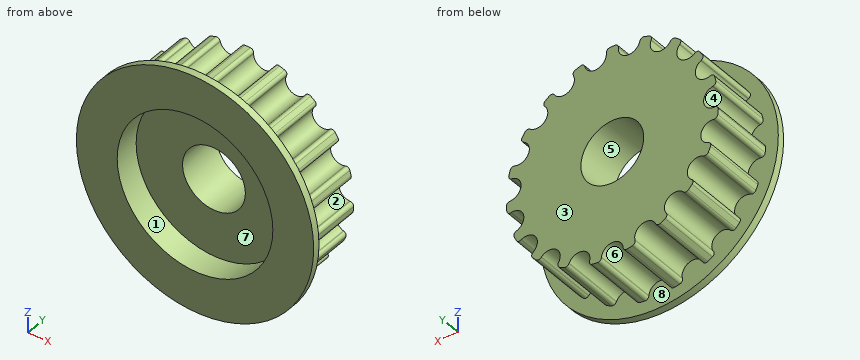
from build123d import *

# Parameters (mm, degrees)
SKETCH_1_R                       = 17
EXTRUDE_1_DEPTH                  = 4.01
SKETCH_3_R                       = 15.205
EXTRUDE_2_DEPTH                  = 9
SKETCH_4_R                       = 4.5
CUT_EXTRUDE_2_DEPTH              = 14.01
CUT_EXTRUDE_4_DEPTH              = 9
FILLET_2_R                       = 0.5
PATTERN_CIRCULAR_7_COUNT         = 19
FILLET_2_OF_PATTERN_CIRCULAR_7_R = 0.5
CUT_EXTRUDE_START                = -3
SKETCH_2_R                       = 11.05
CUT_EXTRUDE_5_DEPTH              = 3
SKETCH_6_R                       = 17
CUT_EXTRUDE_6_DEPTH              = 3
SKETCH_7_R                       = 11.15
CUT_EXTRUDE_7_DEPTH              = 3.6


with BuildPart() as part:
    # Sketch 1 → Extrude 1 (new body)
    with BuildSketch(Plane(origin=(0, 0, 0), x_dir=(1, 0, 0), z_dir=(0, 1, 0))):
        Circle(SKETCH_1_R)
    extrude(amount=EXTRUDE_1_DEPTH)

    # Sketch 3 → Extrude 2 (add)
    with BuildSketch(Plane(origin=(0, 4.01, 0), x_dir=(1, 0, 0), z_dir=(0, 1, 0))):
        Circle(SKETCH_3_R)
    extrude(amount=EXTRUDE_2_DEPTH)

    # Sketch 4 → Cut-Extrude 2 (cut, through all)
    with BuildSketch(Plane(origin=(0, 13.01, 0), x_dir=(1, 0, 0), z_dir=(0, 1, 0))):
        Circle(SKETCH_4_R)
    extrude(amount=-CUT_EXTRUDE_2_DEPTH, mode=Mode.SUBTRACT)

    # Sketch 5 → Cut-Extrude 4 (cut)
    with BuildSketch(Plane(origin=(0, 13.01, 0), x_dir=(1, 0, 0), z_dir=(0, 1, 0))):
        with BuildLine():
            Line((-1.615240041, 15.118962418), (-1.551172735, 14.519279917))
            ThreePointArc((-1.551172735, 14.519279917), (-2e-09, 13.125), (1.551172735, 14.519279913))
            Line((1.551172735, 14.519279913), (1.615240041, 15.118962418))
            ThreePointArc((1.615240041, 15.118962418), (0, 15.205), (-1.615240041, 15.118962418))
        make_face()
    cut_extrude_4 = extrude(amount=-CUT_EXTRUDE_4_DEPTH, mode=Mode.SUBTRACT)

    # Fillet 2
    fillet_2_edges = [part.edges().sort_by_distance(p)[0] for p in [
        (-1.615240041, 8.51, -15.118962418),
        (1.615240041, 8.51, -15.118962418),
    ]]
    fillet(fillet_2_edges, radius=FILLET_2_R)

    # Pattern Circular 7: Cut-Extrude 4 ×19 about axis
    pattern_circular_7_axis = Axis((0, 0, 0), (0, 1, 0))
    for i in range(1, PATTERN_CIRCULAR_7_COUNT):
        add(cut_extrude_4.rotate(pattern_circular_7_axis, i * 360 / PATTERN_CIRCULAR_7_COUNT), mode=Mode.SUBTRACT)

    # Fillet 2 of Pattern Circular 7
    fillet_2_of_pattern_circular_7_edges = [part.edges().sort_by_distance(p)[0] for p in [
        (-6.436840952, 8.51, -13.775307748),
        (-3.381397192, 8.51, -14.824242916),
        (-10.560910269, 8.51, -10.938884737),
        (-8.011607571, 8.51, -12.923086672),
        (-13.540541088, 8.51, -6.917063831),
        (-11.773635958, 8.51, -9.621513464),
        (-15.052844177, 8.51, -2.145671729),
        (-14.259808201, 8.51, -5.27729998),
        (-14.933938031, 8.51, 2.858237198),
        (-15.200708962, 8.51, -0.361209156),
        (-13.196707975, 8.51, 7.552411775),
        (-14.494377044, 8.51, 4.594024283),
        (-10.029409842, 8.51, 11.428165348),
        (-12.217354469, 8.51, 9.051423909),
        (-5.775269531, 8.51, 14.065499879),
        (-8.616391966, 8.51, 12.527961306),
        (-0.895289153, 8.51, 15.17861925),
        (-4.081709697, 8.51, 14.646899704),
        (4.081709697, 8.51, 14.646899704),
        (0.895289153, 8.51, 15.17861925),
        (8.616391966, 8.51, 12.527961306),
        (5.775269531, 8.51, 14.065499879),
        (12.217354469, 8.51, 9.051423909),
        (10.029409842, 8.51, 11.428165348),
        (14.494377044, 8.51, 4.594024283),
        (13.196707975, 8.51, 7.552411775),
        (15.200708962, 8.51, -0.361209156),
        (14.933938031, 8.51, 2.858237198),
        (14.259808201, 8.51, -5.27729998),
        (15.052844177, 8.51, -2.145671729),
        (11.773635958, 8.51, -9.621513464),
        (13.540541088, 8.51, -6.917063831),
        (8.011607571, 8.51, -12.923086672),
        (10.560910269, 8.51, -10.938884737),
        (3.381397192, 8.51, -14.824242916),
        (6.436840952, 8.51, -13.775307748),
    ]]
    fillet(fillet_2_of_pattern_circular_7_edges, radius=FILLET_2_OF_PATTERN_CIRCULAR_7_R)

    # Sketch 2 → Cut-Extrude 5 (cut)
    with BuildSketch(Plane.XZ.offset(CUT_EXTRUDE_START)):
        Circle(SKETCH_2_R)
    extrude(amount=CUT_EXTRUDE_5_DEPTH, mode=Mode.SUBTRACT)

    # Sketch 6 → Cut-Extrude 6 (cut)
    with BuildSketch(Plane.XZ):
        Circle(SKETCH_6_R)
    extrude(amount=-CUT_EXTRUDE_6_DEPTH, mode=Mode.SUBTRACT)

    # Sketch 7 → Cut-Extrude 7 (cut)
    with BuildSketch(Plane.XZ.offset(-3)):
        Circle(SKETCH_7_R)
    extrude(amount=-CUT_EXTRUDE_7_DEPTH, mode=Mode.SUBTRACT)


solid = part.part
Could you check a few things on this model? Use its own coordinates, in mm. Face numbers are marked on the shaded views. A direction names the side the tool comes from. Give positions to 0.01 mm unless a question says otherwise; leave off trailing zeros. Order: outer loops, then holes, each group sorted by start corner. A loop starts at its lowest first (then second) coordinate and runs counter-clockwise, first axis right, second up.
1. Will these pins go through, and if not, where does the flat tip stop? P1, Ø1, axis at x = -5.5, y = 7.5, coming from the +Z side; P2, Ø18, axis at x = 0, z = 0, coming from the +Y side; P3, Ø6, axis at y = 11.5, z = 1, coming from the +X side; P4, Ø1, axis at x = -11, y = 5.5, coming from the +Z side.
2. We'd pull the mould along X, two halves only. Please class the marked faces 1, 2 and 3: pulls with the +X half, pulls with the -X half, needs draft (parallel to the pull), parting line crosses it, or undercut.
3. I need wall thicknesses on L1, parallel to Z at x = 0, y = 4.5 (3 decimals); L2, parallel to X at y = 8, z = -13.5; L3, parallel to Y at x = -11, z = -0.5. Which ranges of each line are inside material? Lowest first, please.
4. For the marked faces 4, 5, 6, 7 and 8, which set-ups out of +Z, -Z, +X, -X, +Y, -Y let a thin tool reach every point of the face, with its end or its side?
5. Suppose I cut it at A-A (z = 5.5). List the corners of the cut face in (x, y) for me, plus the area to 3 significant figures.
Solved:
1. P1: stops at z = 14.36
1. P2: stops at y = 13.01
1. P3: stops at x = 15.18
1. P4: stops at z = 8.55
2. face 1: undercut
2. face 2: pulls with the +X half
2. face 3: needs draft
3. L1: z = -13.125 to -11.15, 11.15 to 15.205
3. L2: x = -7 to -6.37, -3.26 to -1.01, 1.01 to 3.26, 6.37 to 7
3. L3: y = 6.6 to 13.01
4. face 4: -X, +Y
4. face 5: +Y, -Y
4. face 6: -Z, +Y
4. face 7: -Y
4. face 8: +Y
5. outline: (-16.09, 3) - (-9.7, 3) - (-9.7, 6.6) - (9.7, 6.6) - (9.7, 3) - (16.09, 3) - (16.09, 4.01) - (11.94, 4.01) - (11.94, 13.01) - (-11.94, 13.01) - (-11.94, 4.01) - (-16.09, 4.01) - close
5. area: 178 mm2
